Work out the finished part from the listing and answer in its coordinate system (mm). A direction names the side the tool comes from. Give positions to 0.01 mm unless a question says otherwise; leave off trailing zeros. Loops run counter-clockwise (first coordinate to the right, second up) from the corner with the lowest first, then second, coordinate; pieces in that order, holes last.
from build123d import *

# Parameters (mm, degrees)
SKETCH_W     = 12
SKETCH_H     = 12
PAD_DEPTH    = 3
SKETCH001_W  = 12.427667
SKETCH001_H  = 57.473638
PAD001_DEPTH = 0.75
SKETCH002_R  = 3
HOLE_DEPTH   = 25


with BuildPart() as part:
    # Sketch → Pad (new body)
    with BuildSketch(Plane.XY):
        with BuildLine():
            Line((-11.5, -60), (-2.5, -60))
            ThreePointArc((-2.5, -60), (-0.732233, -59.267767), (0, -57.5))
            Line((0, -57.5), (0, -2.5))
            ThreePointArc((0, -2.5), (-0.732233, -0.732233), (-2.5, 0))
            Line((-2.5, 0), (-11.5, 0))
            ThreePointArc((-11.5, 0), (-13.267767, -0.732233), (-14, -2.5))
            Line((-14, -2.5), (-14, -57.5))
            ThreePointArc((-14, -57.5), (-13.267767, -59.267767), (-11.5, -60))
        make_face()
        with Locations((-7, -52)):
            Rectangle(SKETCH_W, SKETCH_H, mode=Mode.SUBTRACT)
        with Locations((-7, -30)):
            Rectangle(SKETCH_W, SKETCH_H, mode=Mode.SUBTRACT)
        with Locations((-7, -8)):
            Rectangle(SKETCH_W, SKETCH_H, mode=Mode.SUBTRACT)
    extrude(amount=PAD_DEPTH)

    # Sketch001 (on Face22 of Pad) → Pad001 (join)
    with BuildSketch(Plane.XY.offset(3)):
        with Locations((-6.943834, -29.736819)):
            Rectangle(SKETCH001_W, SKETCH001_H)
    extrude(amount=-PAD001_DEPTH)

    # Sketch002 (on Face23 of Pad001) → Hole (cut)
    with BuildSketch(Plane(origin=(0, 0, 2.25), x_dir=(1, 0, 0), z_dir=(0, 0, -1))):
        with Locations((-7, 30)):
            Circle(SKETCH002_R)
        with Locations((-7, 52)):
            Circle(SKETCH002_R)
        with Locations((-7, 8)):
            Circle(SKETCH002_R)
    extrude(amount=-HOLE_DEPTH, mode=Mode.SUBTRACT)


solid = part.part
Item 1: A flat-ended cylindrical pin translates along its axis: pin 1 Ø7 at (x, y) = (-7, -30) entering from -Z. Find the tip coordinate at first contact, or state that the pin passes through.
Item 2: Find section A-A, the plane x = -7. Write down the section's boundary in (y, z), plus the area to 3 significant figures.
Item 3: Consider line 1 (Y direction, x = -7, z = 2.75); line 2 (Y direction, x = -8.5, z = 1.3); line 3 (X direction, y = -8, z = 2.6). Determine where each line is inside the solid, lowest interval first.
Item 4: Find section B-B, the plane z = 1.7. Write down the section's boundary in (x, y).
Item 5: Determine the mould class of faces 1 (the face through (-1, -8, 1)), 2 (the face through (-14, -30, 1)), 3 (the face through (-0.752, -59.287, 1.479)) for opening direction Y: released by +Y, released by -Y, zero draft, split by the parting line, or undercut.
Item 6: For faces 4 (the face through (-7, -58, 1)), 5 (the face through (-13.248, -0.713, 1.479)), determine the directions among +Z, -Z, +X, -X, +Y, -Y from which every point of the face is accessible in a straight line to the end or side of a thin tool.
Item 7: Find section D-D, the plane y = -55.5. Write down the section's boundary in (x, z), plus the area to 3 significant figures.
Item 8: Find section C-C, the plane y = -30. Write down the section's boundary in (x, z), plus the area to 3 significant figures.
Ans:
1. pin 1: stops at z = 2.25
2. outline: (-60, 0) - (-58, 0) - (-58, 2.25) - (-55, 2.25) - (-55, 3) - (-60, 3) - close; (-49, 2.25) - (-46, 2.25) - (-46, 0) - (-36, 0) - (-36, 2.25) - (-33, 2.25) - (-33, 3) - (-49, 3) - close; (-27, 2.25) - (-24, 2.25) - (-24, 0) - (-14, 0) - (-14, 2.25) - (-11, 2.25) - (-11, 3) - (-27, 3) - close; (-5, 2.25) - (-2, 2.25) - (-2, 0) - (0, 0) - (0, 3) - (-5, 3) - close
2. area: 85.5 mm2
3. line 1: y = -60 to -55, -49 to -33, -27 to -11, -5 to 0
3. line 2: y = -60 to -58, -46 to -36, -24 to -14, -2 to 0
3. line 3: x = -14 to -10, -4 to 0
4. outline: (-14, -57.5) arc R2.5 ccw to (-11.5, -60) - (-2.5, -60) arc R2.5 ccw to (0, -57.5) - (0, -2.5) arc R2.5 ccw to (-2.5, 0) - (-11.5, 0) arc R2.5 ccw to (-14, -2.5) - close; hole (-13, -58) - (-1, -58) - (-1, -46) - (-13, -46) - close; hole (-13, -36) - (-1, -36) - (-1, -24) - (-13, -24) - close; hole (-13, -14) - (-1, -14) - (-1, -2) - (-13, -2) - close
5. face 1: undercut
5. face 2: zero draft
5. face 3: released by -Y
6. face 4: -Z
6. face 5: +Z, -Z, -X, +Y
7. outline: (-14, 0) - (-13, 0) - (-13, 2.25) - (-1, 2.25) - (-1, 0) - (0, 0) - (0, 3) - (-14, 3) - close
7. area: 15.0 mm2
8. outline: (-14, 0) - (-13, 0) - (-13, 2.25) - (-10, 2.25) - (-10, 3) - (-14, 3) - close; (-4, 2.25) - (-1, 2.25) - (-1, 0) - (0, 0) - (0, 3) - (-4, 3) - close
8. area: 10.5 mm2
